The listing builds one solid part. Answer for the finished solid, in the listing's coordinates (mm). A direction names the side the tool comes from. Coordinates: 2 decimals unless noted, no trailing zeros. Loops run counter-clockwise (first coordinate to the right, second up) from the corner with the lowest first, then second, coordinate; pieces in that order, holes last. Notation, with made-up numbers: (68, 26) - (127, 26) arc R35 ccw to (127, 58) - close; hole circle Ø10 at (-10.75, 35). An arc over 180 degrees is marked (long way). Write each question's results on one line, items separated by ' | '. Start each with the question number.
(1) For faces 1 (the flat face through (-50, 1, -1)), 2 (the flat face through (-65, 2, -13.815)), 3 (the flat face through (-13, 1, -3)), 4 (the flat face through (-20, 2, -38)), 5 (the flat face through (-62, 1, -72)), determine the directions among +Z, -Z, +X, -X, +Y, -Y from which every point of the face is accessible in a straight line to the end or side of a thin tool.
(2) Consider line 1 (Z direction, x = -37.5, y = 2.1); line 2 (Z direction, x = -67.5, y = 2.2); line 3 (X direction, y = 2.4, z = -1.5). Determine where each line is inside the solid, lowest interval first. Write a range as from..to.
(3) Find section D-D on y = 1.6. State how many separate pieces and enclosed holes the cut face has, then the cut area to 3 significant figures.
(4) Find section B-B on z = -73.5. Determine the outline of the cut face in (x, y), then the cut area to 3 significant figures.
(5) Determine the mould class of faces 6 (the cylindrical face through (-37.695, 1.479, -72.013)), 7 (the flat face through (-10, 2, -61.185)), 8 (the flat face through (-25, 1, -1)) for opening direction X: released by +X, released by -X, zero draft, split by the parting line, or undercut.
(6) Find section C-C on x = -58.5. Determine the outline of the cut face in (y, z), then the cut area to 3 significant figures.
(7) Find section A-A on x = -37.5. Determine the outline of the cut face in (y, z), then the cut area to 3 significant figures.
(8) Given pin 1 Ø1 at (x, y) = (-54.5, 0.5) entering from +Z; pin 2 Ø0.9 at (y, z) = (1, -73.5) entering from +X; pin 3 Ø1.5 at (y, z) = (1, -26.5) entering from +X, each flat-ended and moving along its own axis, determine where each tip first touches the part or whether it passes through.
Autodesk Inventor part; units mm, degrees
ref_plane "YZ Plane" through (0, 0, 0) normal (1, 0, 0) x (0, 1, 0)
ref_plane "XZ Plane" through (0, 0, 0) normal (0, 1, 0) x (-1, 0, 0)
ref_plane "XY Plane" through (0, 0, 0) normal (0, 0, 1) x (1, 0, 0)
sketch "Sketch1" plane through (0, 0, 0) normal (0, 1, 0) x (-1, 0, 0)
  line L0 (25, 0) -> (50, 0)
  line L1 (50, -75) -> (25, -75)
  line L2 (75, 0) -> (75, -25)
  line L3 (75, -25) -> (72, -25)
  line L4 (75, -75) -> (75, -50)
  line L5 (75, -50) -> (72, -50)
  line L6 (72, -50) -> (72, -25)
  line L7 (0, -25) -> (3, -25)
  line L8 (3, -25) -> (3, -50)
  line L9 (3, -50) -> (0, -50)
  line L10 (0, -75) -> (3, -75)
  line L11 (25, -75) -> (25, -72)
  line L12 (25, -72) -> (0, -72)
  line L13 (75, -75) -> (72, -75)
  line L14 (50, -75) -> (50, -72)
  line L15 (50, -72) -> (75, -72)
  line L16 (50, 0) -> (50, -3)
  line L17 (50, -3) -> (75, -3)
  line L18 (25, 0) -> (25, -3)
  line L19 (25, -3) -> (0, -3)
  line L20 (75, 0) -> (75, -25)
  line L21 (75, -50) -> (75, -75)
  line L22 (0, -75) -> (0, -50)
  line L23 (0, -25) -> (0, 0)
  dimension "d0" = 75
  dimension "d1" = 75
  dimension "d2" = 25
  dimension "d3" = 3
  dimension "d4" = 25
  dimension "d5" = 3
  dimension "d6" = 25
  dimension "d7" = 3
  dimension "d8" = 25
  dimension "d9" = 3
  dimension "d10" = 3
extrude "Extrusion1" add sketch "Sketch1" along normal blind 3
sketch "Sketch3" plane through (0, 0, 0) normal (0, -1, 0) x (1, 0, 0)
  line L0 (-3, -13.8146) -> (0, -13.8146)
  line L1 (0, -61.1854) -> (-3, -61.1854)
  line L2 (-72, -61.1854) -> (-75, -61.1854)
  line L3 (-75, -13.8146) -> (-72, -13.8146)
  line L4 (0, -61.1854) -> (-20, -61.1854)
  line L5 (-20, -61.1854) -> (-20, -13.8146)
  line L6 (0, -13.8146) -> (-20, -13.8146)
  line L7 (-75, -13.8146) -> (-55, -13.8146)
  line L8 (-55, -13.8146) -> (-55, -61.1854)
  line L9 (-75, -61.1854) -> (-55, -61.1854)
  line L10 (-75, -61.1854) -> (-75, -13.8146)
  line L11 (0, -13.8146) -> (0, -61.1854)
  line L12 (0, -50) -> (0, -72)
  point P0 (0, 0)
  dimension "d13" = 20
  dimension "d14" = 20
extrude "Extrusion2" cut sketch "Sketch3" along normal mid plane 25.4
sketch "Sketch4" plane through (0, 0, 0) normal (0, -1, 0) x (1, 0, 0)
  circle A0 centre (-30.7671, -9.9986) radius 1.14
  circle A1 centre (-44.2271, -10.0014) radius 1.14
  arc A2 (-31.5, -28.5) -> (-33.5, -28.5) centre (-32.5, -28.5) ccw
  circle A3 centre (-30.7671, -64.9995) radius 1.14
  circle A4 centre (-44.2271, -65.0005) radius 1.14
  arc A5 (-41.5, -28.5) -> (-43.5, -28.5) centre (-42.5, -28.5) ccw
  circle A6 centre (-42.5, -28.5) radius 1
  circle A7 centre (-32.5, -28.5) radius 1
  circle A8 centre (-30.7671, -64.9995) radius 1.14
  circle A9 centre (-44.2271, -65.0005) radius 1.14
  circle A10 centre (-44.2271, -10.0014) radius 1.14
  circle A11 centre (-30.7671, -9.9986) radius 1.14
  arc A12 (-33.5, -46.5) -> (-31.5, -46.5) centre (-32.5, -46.5) ccw
  arc A13 (-43.5, -46.5) -> (-41.5, -46.5) centre (-42.5, -46.5) ccw
  circle A14 centre (-32.5, -46.5) radius 1
  circle A15 centre (-42.5, -46.5) radius 1
  point P0 (0, 0)
extrude "Extrusion3" cut sketch "Sketch4" against normal blind 3 contours A0 | A1 | A3 | A4
sketch "Sketch5" plane through (0, 0, 0) normal (0, -1, 0) x (1, 0, 0)
  line L0 (-17.5, -6) -> (-17.5, -17)
  line L1 (-17.5, -17) -> (-29.5, -17)
  line L2 (-47, -17) -> (-56, -17)
  line L3 (-56, -6) -> (-56, -17)
  line L4 (-17.5, -17) -> (-29.5, -17)
  line L5 (-29.5, -17) -> (-29.5, -6)
  line L6 (-29.5, -6) -> (-17.5, -6)
  line L7 (-17.5, -6) -> (-17.5, -17)
  line L8 (-56, -17) -> (-47, -17)
  line L9 (-47, -17) -> (-47, -6)
  line L10 (-47, -6) -> (-56, -6)
  line L11 (-56, -6) -> (-56, -17)
  arc A0 (-23.098, -46.5011) -> (-21.098, -46.5011) centre (-22.098, -46.5011) ccw
  circle A1 centre (-22.098, -28.5012) radius 1
  arc A2 (-21.098, -28.5011) -> (-23.098, -28.5011) centre (-22.098, -28.5011) ccw
  arc A3 (-23.098, -46.5011) -> (-21.098, -46.5011) centre (-22.098, -46.5011) ccw
  circle A4 centre (-22.098, -46.5078) radius 1
  line L12 (-72, -25) -> (-72, -3)
  line L13 (-25, -3) -> (-3, -3)
  line L14 (-50, -72) -> (-72, -72)
  circle A5 centre (-52.902, -46.4986) radius 1
  arc A6 (-51.902, -28.4986) -> (-53.902, -28.4986) centre (-52.902, -28.4986) ccw
  circle A7 centre (-52.902, -28.492) radius 1
  circle A8 centre (-37.5, -1.5) radius 1.5
  circle A9 centre (-1.5, -37.5) radius 1.5
  circle A10 centre (-37.5, -73.5) radius 1.5
  circle A11 centre (-73.5, -36) radius 1.5
  circle A12 centre (-73.5, -36) radius 1.5
  circle A13 centre (-73.5, -36) radius 1.5
  circle A14 centre (-37.5, -1.5) radius 1.5
  circle A15 centre (-37.5, -73.5) radius 1.5
  circle A16 centre (-37.5, -73.5) radius 1.5
  line L15 (-72, -50) -> (-75, -50)
  circle A17 centre (-37.5, -73.5) radius 1.5
  circle A18 centre (-37.5, -73.5) radius 1.5
  circle A19 centre (-37.5, -73.5) radius 1.5
  circle A20 centre (-37.5, -73.5) radius 1.5
  circle A21 centre (-37.5, -73.5) radius 1.5
  circle A22 centre (-37.5, -73.5) radius 1.5
  circle A23 centre (-37.5, -73.5) radius 1.5
  circle A24 centre (-37.5, -73.5) radius 1.5
  circle A25 centre (-37.5, -73.5) radius 1.5
  circle A26 centre (-37.5, -73.5) radius 1.5
  circle A27 centre (-37.5, -73.5) radius 1.5
  circle A28 centre (-37.5, -73.5) radius 1.5
  circle A29 centre (-37.5, -1.5) radius 1.5
  circle A30 centre (-37.5, -73.5) radius 1.5
  circle A31 centre (-37.5, -73.5) radius 1.5
  circle A32 centre (-36.0014, -62.75) radius 1.5
  line L16 (-50, -72) -> (-50, -75.5)
  line L17 (-72, -72) -> (-72, -50)
  line L18 (-75, -50) -> (-75, -25)
  line L19 (-75, -25) -> (-72, -25)
  line L20 (-72, -3) -> (-50, -3)
  line L21 (-50, -3) -> (-50, 0.5)
  line L22 (-25, 0.5) -> (-50, 0.5)
  line L23 (-25, -3) -> (-25, 0.5)
  line L24 (-3, -3) -> (-3, -25)
  line L25 (-3, -25) -> (0, -25)
  line L26 (0, -25) -> (0, -50)
  line L27 (0, -50) -> (-3, -50)
  line L28 (-3, -50) -> (-3, -72)
  line L29 (-3, -72) -> (-25, -72)
  line L30 (-25, -72) -> (-25, -75.5)
  line L31 (-50, -75.5) -> (-25, -75.5)
  point P0 (0, 0)
  point P1 (-37.5, -1.5)
  point P2 (-37.5, 0)
extrude "Extrusion4" cut sketch "Sketch5" against normal blind 25.4 contours A4 A0 | A0 A4 | A1 | A5 | A7 A6 | A6 A7
sketch "Sketch6" plane through (0, 0, 0) normal (0, -1, 0) x (1, 0, 0)
  circle A0 centre (-52.902, -46.4986) radius 1
  arc A1 (-21.098, -28.5011) -> (-23.098, -28.5011) centre (-22.098, -28.5011) ccw
  arc A2 (-23.098, -28.5011) -> (-21.098, -28.5011) centre (-22.098, -28.5012) ccw
  circle A3 centre (-22.098, -46.5078) radius 1
  circle A4 centre (-52.902, -28.492) radius 1
  circle A5 centre (-30.7671, -64.9995) radius 1.14
  circle A6 centre (-30.7671, -9.9986) radius 1.14
  circle A7 centre (-44.2271, -10.0014) radius 1.14
  circle A8 centre (-44.2271, -65.0005) radius 1.14
  line L0 (0, -61.1854) -> (-20, -61.1854)
  line L1 (-20, -61.1854) -> (-20, -13.8146)
  line L2 (-20, -13.8146) -> (0, -13.8146)
  line L3 (0, -3) -> (0, -13.8146)
  line L4 (-25, -3) -> (0, -3)
  line L5 (-25, 0) -> (-25, -3)
  line L6 (-50, 0) -> (-25, 0)
  line L7 (-50, -3) -> (-50, 0)
  line L8 (-75, -3) -> (-50, -3)
  line L9 (-75, -13.8146) -> (-75, -3)
  line L10 (-75, -13.8146) -> (-55, -13.8146)
  line L11 (-55, -13.8146) -> (-55, -61.1854)
  line L12 (-55, -61.1854) -> (-75, -61.1854)
  line L13 (-75, -72) -> (-75, -61.1854)
  line L14 (-50, -72) -> (-75, -72)
  line L15 (-50, -75) -> (-50, -72)
  line L16 (-25, -75) -> (-50, -75)
  line L17 (-25, -72) -> (-25, -75)
  line L18 (0, -72) -> (-25, -72)
  line L19 (0, -61.1854) -> (0, -72)
  circle A9 centre (-37.5, -73.5) radius 1.5
  circle A10 centre (-37.5, -1.5) radius 1.5
  point P0 (0, 0)
  dimension "d21" = 3
  dimension "d25" = 3
extrude "Extrusion5" cut sketch "Sketch6" against normal blind 25.4 contours A10 | A9
sketch "Sketch7" plane through (-50, 0, 0) normal (0, 0, 1) x (1, 0, 0)
  line L0 (12.5, 0) -> (12.5, 3)
  line L1 (12.5, 0) -> (25, 0)
  line L2 (25, 0) -> (25, 3)
  line L3 (12.5, 3) -> (25, 3)
  line L4 (0, 3) -> (12.5, 3)
  line L5 (0, 0) -> (0, 3)
  line L6 (0, 0) -> (12.5, 0)
  line L7 (12.5, 0) -> (12.5, 3)
  line L8 (0, 3) -> (12.5, 3)
  line L9 (0, 0) -> (0, 3)
  line L10 (0, 0) -> (12.5, 0)
  line L11 (12.5, 0) -> (25, 0)
  line L12 (25, 0) -> (25, 3)
  line L13 (12.5, 3) -> (25, 3)
  point P0 (50, 0)
extrude "Extrusion6" add sketch "Sketch7" along normal blind 0.5
sketch "Sketch8" plane through (-50, 0, -75) normal (0, 0, -1) x (-1, 0, 0)
  line L0 (0, 0) -> (-25, 0)
  line L1 (-25, 0) -> (-25, 3)
  line L2 (-25, 3) -> (0, 3)
  line L3 (0, 3) -> (0, 0)
  point P0 (-50, 0)
extrude "Extrusion7" add sketch "Sketch8" along normal blind 0.5
properties part number "Base"
Values:
1) face 1: +Z, -X, +Y, -Y | face 2: -X, +Y, -Y | face 3: +Z, +X, +Y, -Y | face 4: +X, +Y, -Y | face 5: -Z, -X, +Y, -Y
2) line 1: z = -75.5..-75, -72..-3, 0..0.5 | line 2: z = -72..-61.19, -13.81..-3 | line 3: x = -50..-39, -36..-25
3) separate pieces: 1 | enclosed holes: 10 | area: 3,410 mm²
4) outline: (-50, 0) - (-39, 0) - (-39, 3) - (-50, 3) - close; (-36, 0) - (-25, 0) - (-25, 3) - (-36, 3) - close | area: 66.0 mm²
5) face 6: undercut | face 7: zero draft | face 8: released by +X
6) outline: (0, -72) - (3, -72) - (3, -61.19) - (0, -61.19) - close; (0, -13.81) - (3, -13.81) - (3, -3) - (0, -3) - close | area: 64.9 mm²
7) outline: (0, -75.5) - (3, -75.5) - (3, -75) - (0, -75) - close; (0, -72) - (3, -72) - (3, -3) - (0, -3) - close; (0, 0) - (3, 0) - (3, 0.5) - (0, 0.5) - close | area: 210 mm²
8) pin 1: stops at z = -3 | pin 2: stops at x = -25 | pin 3: stops at x = -20
